Build history of the part. All positions in model axes, mm. Coordinates: 2 decimals unless noted, no trailing zeros. Order: outer loops, then holes, each group sorted by start corner. A loop starts at its lowest first (then second) coordinate and runs counter-clockwise, first axis right, second up. Notation, with made-up numbers: (23, 66.25) -> (71, 66.25) arc R22 ccw to (71, 78.25) -> close; hole circle Ø10 at (87, -36.75). An arc over 180 degrees is marked (long way). Write each question's results on one line, items separated by ' | '.
from build123d import *

# Parameters (mm, degrees)
F0_R     = 12.5
F0_R_2   = 9.5
F1_DEPTH = 25
F2_W     = 68.842221
F2_H     = 15.526487
F3_DEPTH = 25


with BuildPart() as f1:
    # F0 (on Top) → F1 (new body)
    with BuildSketch(Plane.XY):
        with BuildLine():
            Line((15.099982, 11.984992), (-15.227959, 14.826929))
            Line((-15.227959, 14.826929), (-16.977903, 14.990911))
            ThreePointArc((-16.977903, 14.990911), (-32.492809, 0.464415), (-17.906726, -14.994485))
            Line((-17.906726, -14.994485), (-14.372817, -14.670403))
            Line((-14.372817, -14.670403), (14.782548, -11.996673))
            ThreePointArc((14.782548, -11.996673), (26.498949, -0.158824), (15.099982, 11.984992))
        make_face()
        with Locations((-17.5, 0)):
            Circle(F0_R, mode=Mode.SUBTRACT)
        with Locations((14.5, 0)):
            Circle(F0_R_2, mode=Mode.SUBTRACT)
    extrude(amount=F1_DEPTH)

    # F2 (on Top) → F3 (cut)
    with BuildSketch(Plane.XY):
        with Locations((-1.820405, -7.763243)):
            Rectangle(F2_W, F2_H)
    extrude(amount=F3_DEPTH, mode=Mode.SUBTRACT)


solid = f1.part
Item 1: Slice it at C-C, the plane x = 14.5. List the corners of the cut face in (y, z), and give its area (3 significant figures).
Answer:
outline: (9.5, 0) -> (12.04, 0) -> (12.04, 25) -> (9.5, 25) -> close | area: 63.5 mm^2
Item 2: Drill centre lines: line 1 (X direction, y = 8.75, z = 16); line 2 (X direction, y = 5.75, z = 13); line 3 (Y direction, x = 21.5, z = 6.75). Where is each one in solid material? Low to high. Write a range as from..to.
Answer:
line 1: x = -29.68..-26.43, -8.57..10.8, 18.2..22.71 | line 2: x = -31.35..-28.6, -6.4..6.94, 22.06..25.03 | line 3: y = 6.42..9.75
Item 3: Pin check, flat tips, straight feed: pin 1 (10 mm diameter, centred on x = 19, z = 13, fed in from +Y); pin 2 (2 mm diameter, centred on x = -21, z = 3.5, fed in from +Y); pin 3 (1.5 mm diameter, centred on y = 6, z = 8.5, fed in from +X). Stop position of each tip, or through.
Answer:
pin 1: stops at y = 12.09 | pin 2: stops at y = 14.79 | pin 3: stops at x = 25.29
Item 4: Slice it at A-A, the plane y = 1. List the corners of the cut face in (x, z).
Answer:
outline: (-32.47, 0) -> (-29.96, 0) -> (-29.96, 25) -> (-32.47, 25) -> close; (-5.04, 0) -> (5.05, 0) -> (5.05, 25) -> (-5.04, 25) -> close; (23.95, 0) -> (26.46, 0) -> (26.46, 25) -> (23.95, 25) -> close
Item 5: Slice it at B-B, the plane z = 2.25. List the corners of the cut face in (x, y) (3 decimals).
Answer:
outline: (-32.5, 0) -> (-30, 0) arc R12.5 cw to (-5, 0) -> (5, 0) arc R9.5 cw to (24, 0) -> (26.5, 0) arc R12 ccw to (15.1, 11.985) -> (-15.228, 14.827) -> (-16.978, 14.991) arc R15 ccw to start
Item 6: Pull direction X, two halves, no side cores. Call faces 1 (the cylindrical face through (23.28, 8.18, 12.32)), 2 (the flat face through (0, 0, 12)), 3 (the cylindrical face through (-17.225, 12.497, 12.325)): released by +X, released by -X, zero draft, split by the parting line, or undercut.
Answer:
face 1: released by +X | face 2: zero draft | face 3: undercut
Item 7: Slice it at D-D, the plane y = 6.5. List the corners of the cut face in (x, z).
Answer:
outline: (-31.02, 0) -> (-28.18, 0) -> (-28.18, 25) -> (-31.02, 25) -> close; (-6.82, 0) -> (7.57, 0) -> (7.57, 25) -> (-6.82, 25) -> close; (21.43, 0) -> (24.59, 0) -> (24.59, 25) -> (21.43, 25) -> close
